Geometry: final body of the model. Coordinates: model frame, mm. A direction names the side the tool comes from. Give positions to 0.01 mm unless a question says otherwise; leave off trailing zeros. Write each loop counter-clockwise with the first axis right and the second up, starting at its lowest first coordinate (ties: lowest second). Pieces come first, ordered by that corner, then holes. Notation, with made-up numbers: M 51,65.25 L 72,65.25 A30 ccw 72,102.25 Z; hole C 2,4.5 d10. An arc over 180 degrees is marked long. Use a Markdown table: item, result. Add a question column.
1) Draft query along X for faces 3 (the flat face through (15, 0, 16)), 4 (the flat face through (0, 14, 16)), 5 (the flat face through (5.726, 7.805, 15.653)), 6 (the cylindrical face through (23.08, 1.97, 25.55)). Return one class per face: +X half, -X half, draft (parallel to the pull), parting line (faces both ways), or undercut.
2) Section A-A on x = 20.4. Return the cut outline in (y, z).
3) Section B-B on z = 9.5. Return the cut outline in (x, y), then the cut area to 3 significant figures.
4) Set-up query: faces 1 (the flat face through (18, 4, 16)), 2 (the flat face through (5, 8, 0)). Return all of +Z, -Z, +X, -X, +Y, -Y with unobstructed straight access to the full face (end or side cutting, diameter ignored); none if empty.
5) Line query: line 1 (Z direction, x = 20.4, y = 1.8); line 2 (Z direction, x = 16, y = 2.1); line 3 (Y direction, x = 8.5, z = 29). Output: solid intervals per line, ascending.
6) Section D-D on y = 19. Return the cut outline in (x, z), then the cut area to 3 significant figures.
7) Section C-C on z = 16.5. Return the cut outline in (x, y), then the cut area to 3 significant figures.
8) Pin query (flat end, axial travel): pin 1 (3 mm diameter, centred on x = 19.5, z = 14.5, fed in from +Y); pin 2 (8 mm diameter, centred on y = 24, z = 6.5, fed in from +X); pin 3 (1.5 mm diameter, centred on x = 9.5, y = 5.5, fed in from +Z). Return the tip coordinate at first contact, or that it passes through.
```python
from build123d import *

# Parameters (mm, degrees)
BOSS_EXTRUDE1_DEPTH     = 31.75
F_1_4_CLEARANCE_HOLE1_D = 6.7564
CHAMFER1_SIZE           = 3.5
CHAMFER1_SIZE2          = 7.505774222


with BuildPart() as part:
    # Sketch1 → Boss-Extrude1 (new body)
    with BuildSketch(Plane.XY):
        Polygon((0, 0), (0, 29.4), (4, 29.4), (4, 4), (29.4, 4), (29.4, 0), align=None)
    extrude(amount=BOSS_EXTRUDE1_DEPTH)

    # 1/4 Clearance Hole1 (through all)
    with Locations(Plane(origin=(0, 4, 0), x_dir=(1, 0, 0), z_dir=(0, 1, 0))):
        with Locations((20.4, -23.495), (16, -8.255)):
            Hole(F_1_4_CLEARANCE_HOLE1_D / 2)

    # Chamfer1
    chamfer1_edges = [part.edges().sort_by_distance(p)[0] for p in [
        (4, 4, 15.875),
    ]]
    chamfer1_side = [part.faces().sort_by_distance(p)[0] for p in [
        (16.553612055, 4, 15.875),
    ]]
    chamfer(chamfer1_edges, length=CHAMFER1_SIZE, length2=CHAMFER1_SIZE2, reference=chamfer1_side[0])


solid = part.part
```
Found:
| question | item | result |
|---|---|---|
| 1 | face 3 | draft |
| 1 | face 4 | -X half |
| 1 | face 5 | +X half |
| 1 | face 6 | undercut |
| 2 | outline | M 0,0 L 4,0 L 4,20.12 L 0,20.12 Z; M 0,26.87 L 4,26.87 L 4,31.75 L 0,31.75 Z |
| 3 | outline | M 0,0 L 12.86,0 L 12.86,4 L 7.5,4 L 4,11.51 L 4,29.4 L 0,29.4 Z; M 19.14,0 L 29.4,0 L 29.4,4 L 19.14,4 Z |
| 3 | area | 207 mm² |
| 4 | face 1 | +Z, -Z, +X, +Y |
| 4 | face 2 | -Z, +X, -X, +Y, -Y |
| 5 | line 1 | 0 to 20.12, 26.87 to 31.75 |
| 5 | line 2 | 0 to 4.88, 11.63 to 31.75 |
| 5 | line 3 | 0 to 4 |
| 6 | outline | M 0,0 L 4,0 L 4,31.75 L 0,31.75 Z |
| 6 | area | 127 mm² |
| 7 | outline | M 0,0 L 29.4,0 L 29.4,4 L 7.5,4 L 4,11.51 L 4,29.4 L 0,29.4 Z |
| 7 | area | 232 mm² |
| 8 | pin 1 | y = 4 |
| 8 | pin 2 | x = 4 |
| 8 | pin 3 | through |
